Read the model definition and answer for the solid it produces. Units are mm, in the model's axes. Give positions to 0.01 mm unless a question says otherwise; leave off trailing zeros. Write each loop counter-clockwise with the first axis right and the second up, starting at its lowest first coordinate (ties: lowest second). Pieces come first, ordered by that corner, then holes.
```python
from build123d import *

# Parameters (mm, degrees)
BOSS_EXTRUDE1_DEPTH = 36.4
CUT_EXTRUDE1_REACH  = 4.6
SKETCH2_R           = 1.1
CUT_EXTRUDE3_START  = -2.6
SKETCH4_W           = 2
SKETCH4_H           = 12
CUT_EXTRUDE3_DEPTH  = 2.6


with BuildPart() as part:
    # Sketch1 → Boss-Extrude1 (new body, symmetric)
    with BuildSketch(Plane.XY):
        Polygon((0, 2.6), (0, 0), (2, 0), (2, 0.6), align=None)
    extrude(amount=BOSS_EXTRUDE1_DEPTH, both=True)

    # Cut-Extrude1: up to this face of the body (flat: up to its plane)
    cut_extrude1_end = Plane(part.part.faces().sort_by_distance((1, 1.6, 0))[0])
    # Sketch2 → Cut-Extrude1 (cut, up to the picked face)
    with BuildSketch(Plane.XZ, mode=Mode.PRIVATE) as cut_extrude1_sk1:
        with Locations((2.2, 0)):
            Circle(SKETCH2_R)
    cut_extrude1_tool1 = split(extrude(cut_extrude1_sk1.sketch, amount=-CUT_EXTRUDE1_REACH, mode=Mode.PRIVATE), bisect_by=cut_extrude1_end, keep=Keep.BOTH, mode=Mode.PRIVATE)
    add(cut_extrude1_tool1.solids().sort_by_distance((2.2, 0, 0))[0], mode=Mode.SUBTRACT)
    # Sketch2 → Cut-Extrude1 (cut, up to the picked face)
    with BuildSketch(Plane.XZ, mode=Mode.PRIVATE) as cut_extrude1_sk2:
        with Locations((2.2, 22)):
            Circle(SKETCH2_R)
    cut_extrude1_tool2 = split(extrude(cut_extrude1_sk2.sketch, amount=-CUT_EXTRUDE1_REACH, mode=Mode.PRIVATE), bisect_by=cut_extrude1_end, keep=Keep.BOTH, mode=Mode.PRIVATE)
    add(cut_extrude1_tool2.solids().sort_by_distance((2.2, 0, 22))[0], mode=Mode.SUBTRACT)
    # Sketch2 → Cut-Extrude1 (cut, up to the picked face)
    with BuildSketch(Plane.XZ, mode=Mode.PRIVATE) as cut_extrude1_sk3:
        with Locations((2.2, -22)):
            Circle(SKETCH2_R)
    cut_extrude1_tool3 = split(extrude(cut_extrude1_sk3.sketch, amount=-CUT_EXTRUDE1_REACH, mode=Mode.PRIVATE), bisect_by=cut_extrude1_end, keep=Keep.BOTH, mode=Mode.PRIVATE)
    add(cut_extrude1_tool3.solids().sort_by_distance((2.2, 0, -22))[0], mode=Mode.SUBTRACT)

    # Sketch4 → Cut-Extrude3 (cut)
    with BuildSketch(Plane(origin=(0, 0, 0), x_dir=(-1, 0, 0), z_dir=(0, -1, 0)).offset(CUT_EXTRUDE3_START)):
        with Locations((-1, 30.4)):
            Rectangle(SKETCH4_W, SKETCH4_H)
    extrude(amount=CUT_EXTRUDE3_DEPTH, mode=Mode.SUBTRACT)


solid = part.part
```
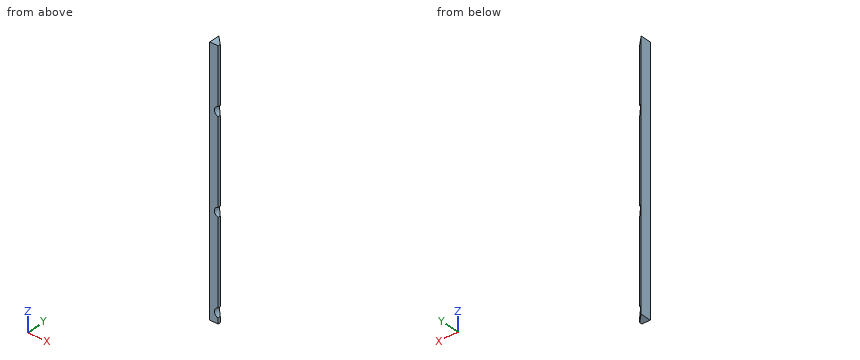
Item 1: Section A-A (x = 1.65) is taken. Write down the section's boundary in (y, z), and give its area (3 significant figures).
Result set:
outline: (0, -24.4) - (0.95, -24.4) - (0.95, -22.95) - (0, -22.95) - close; (0, -21.05) - (0.95, -21.05) - (0.95, -0.95) - (0, -0.95) - close; (0, 0.95) - (0.95, 0.95) - (0.95, 21.05) - (0, 21.05) - close; (0, 22.95) - (0.95, 22.95) - (0.95, 36.4) - (0, 36.4) - close
area: 52.3 mm2
Item 2: Section C-C (z = -5) is taken. Write down the section's boundary in (x, y), and give its area (3 significant figures).
Result set:
outline: (0, 0) - (2, 0) - (2, 0.6) - (0, 2.6) - close
area: 3.20 mm2
Item 3: Section B-B (y = 1.05) is taken. Write down the section's boundary in (x, z), and give its area (3 significant figures).
Result set:
outline: (0, -24.4) - (1.55, -24.4) - (1.55, -22.89) arc R1.1 cw to (1.55, -21.11) - (1.55, -0.89) arc R1.1 cw to (1.55, 0.89) - (1.55, 21.11) arc R1.1 cw to (1.55, 22.89) - (1.55, 36.4) - (0, 36.4) - close
area: 92.6 mm2
Item 4: Find the intervals of material crossed by line 1 along X through (y, z) = (2.25, 6); line 2 along Y through (x, z) = (0.15, -15.5); line 3 along Y through (x, z) = (1.95, 3.5), in increasing order.
Result set:
line 1: x = 0 to 0.35
line 2: y = 0 to 2.45
line 3: y = 0 to 0.65
